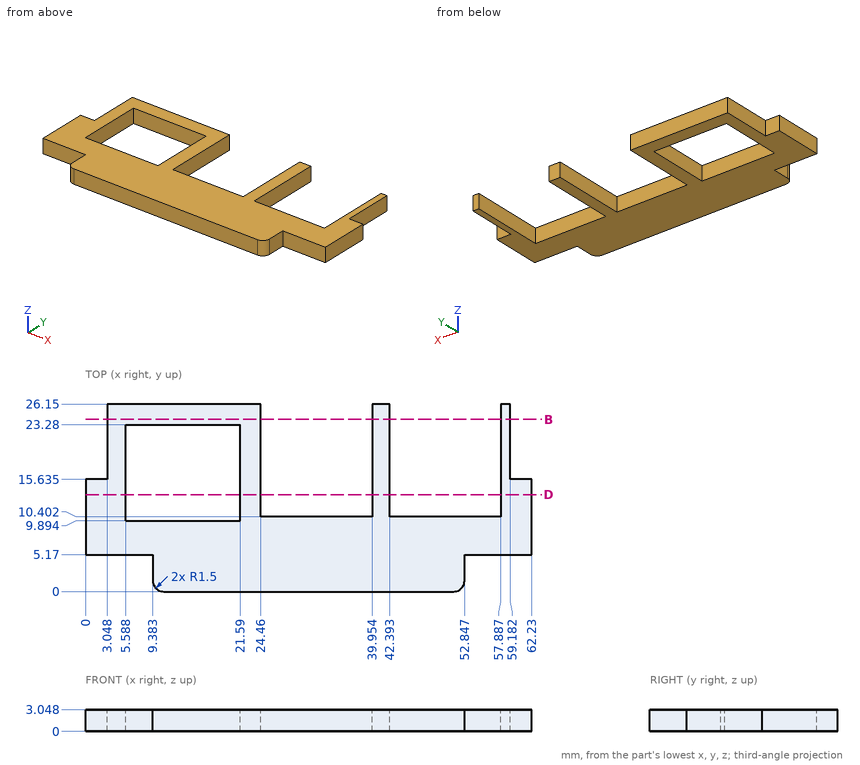
The figure shows three views and two pictorial views of one solid part (mm, origin at its lowest corner). Answer the questions. Round coordinates to 2 decimals unless told otherwise and drop trailing zeros. Write each loop counter-clockwise with the first axis right and the second up, starting at its lowest first coordinate (ties: lowest second). Pieces come first, ordered by that corner, then holes. Notation, with made-up numbers: (-37, 79.25) -> (-9, 79.25) arc R17 ccw to (-9, 105.25) -> close; hole circle Ø11 at (89.5, 16). An arc over 180 degrees is marked (long way). Write each question's results on one line, items separated by ' | '.
Q1. Section D-D, the plane y = 13.5 is taken. Write down the section's boundary in (x, z) (1 decimal).
Data:
outline: (0, 0) -> (5.6, 0) -> (5.6, 3) -> (0, 3) -> close; (21.6, 0) -> (24.5, 0) -> (24.5, 3) -> (21.6, 3) -> close; (40, 0) -> (42.4, 0) -> (42.4, 3) -> (40, 3) -> close; (57.9, 0) -> (62.2, 0) -> (62.2, 3) -> (57.9, 3) -> close
Q2. Flat-ended cylindrical pins translate along their axes: P1, Ø0.9, axis at y = 3.5, z = 1, coming from the -X side; P2, Ø0.9, axis at y = 4, z = 2, coming from the +X side; P3, Ø3, axis at x = 55.5, y = 19, coming from the +Z side; P4, Ø0.9, axis at x = 61.5, z = 1, coming from the +Y side (1 decimal). Find the tip coordinate at first contact, or state that the pin passes through.
Data:
P1: x = 9.38 | P2: x = 52.85 | P3: through | P4: y = 15.6
Q3. Section B-B, the plane y = 24 is taken. Write down the section's boundary in (x, z) (1 decimal).
Data:
outline: (3, 0) -> (24.5, 0) -> (24.5, 3) -> (3, 3) -> close; (40, 0) -> (42.4, 0) -> (42.4, 3) -> (40, 3) -> close; (57.9, 0) -> (59.2, 0) -> (59.2, 3) -> (57.9, 3) -> close
Q4. Straight lines are drawn through the part: line 1 along X through (y, z) = (15.25, 1.55) (1 decimal); line 2 along X through (y, z) = (24.5, 1.8) (1 decimal); line 3 along X through (y, z) = (18, 1.8) (1 decimal). For each, find the intervals that lie inside material, in ascending order. Write a range as [from, to].
Data:
line 1: [0, 5.6], [21.6, 24.5], [40, 42.4], [57.9, 62.2] | line 2: [3, 24.5], [40, 42.4], [57.9, 59.2] | line 3: [3, 5.6], [21.6, 24.5], [40, 42.4], [57.9, 59.2]
